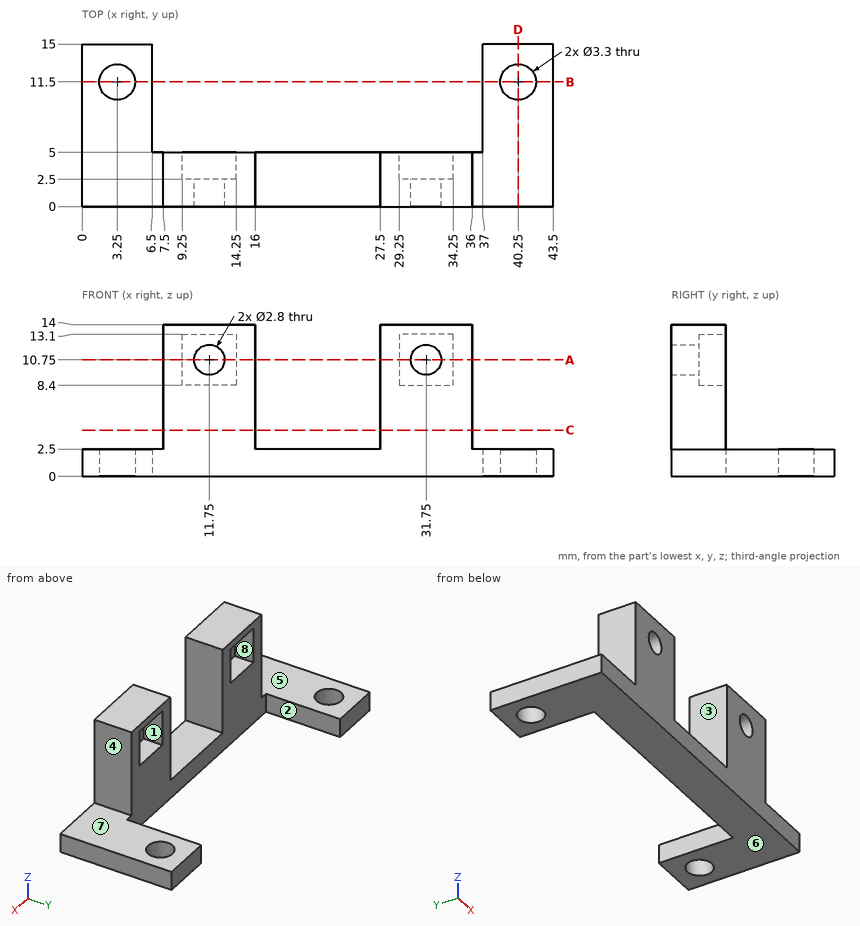
Verification items for this drawing (mm, ordinates from the low corner). A direction names the side the tool comes from. Give positions to 0.01 mm unless a question says otherwise; leave off trailing zeros. Write each loop counter-clockwise with the first axis right and the second up, starting at its lowest first coordinate (ties: lowest second). Pieces come first, ordered by that corner, then holes.
1) Gauge pin test, flat ends, axial feed: pin 1 (5.5 mm diameter, centred on y = 3, z = 10.5, fed in from -X); pin 2 (4.5 mm diameter, centred on x = 31.75, z = 10.75, fed in from +Y); pin 3 (4 mm diameter, centred on y = 2.5, z = 10.5, fed in from +X). Record the tip position at first contact, or that the pin passes through.
2) Section check A-A, the plane z = 10.75. Record the boundary of the cut face in (x, y).
3) Release check for a two-part mould opening along Z. For the marked faces 6, 7 and 8 record: pulls with the +Z half, pulls with the -Z half, needs draft (parallel to the pull), parting line crosses it, or undercut.
4) Material ranges on L1, parallel to X at y = 11.5, z = 0.8; L2, parallel to X at y = 4.75, z = 12; L3, parallel to Z at x = 31, y = 4.25, recorded low to high.
5) Section check C-C, the plane z = 4.25. Record the boundary of the cut face in (x, y), and give its area (3 significant figures).
6) Access from +Z, -Z, +X, -X, +Y, -Y to the whole of each face (thin tool, end or side, straight path). Record for the marked faces 1, 2, 3, 4 and 5.
7) Section check D-D, the plane x = 40.25. Record the boundary of the cut face in (y, z).
8) Section check B-B, the plane y = 11.5. Record the boundary of the cut face in (x, z), and give its area (3 significant figures).
Computed:
1. pin 1: stops at x = 7.5
1. pin 2: stops at y = 2.5
1. pin 3: stops at x = 36
2. outline: (7.5, 0) - (10.35, 0) - (10.35, 2.5) - (9.25, 2.5) - (9.25, 5) - (7.5, 5) - close; (13.15, 0) - (16, 0) - (16, 5) - (14.25, 5) - (14.25, 2.5) - (13.15, 2.5) - close; (27.5, 0) - (30.35, 0) - (30.35, 2.5) - (29.25, 2.5) - (29.25, 5) - (27.5, 5) - close; (33.15, 0) - (36, 0) - (36, 5) - (34.25, 5) - (34.25, 2.5) - (33.15, 2.5) - close
3. face 6: pulls with the -Z half
3. face 7: pulls with the +Z half
3. face 8: undercut
4. L1: x = 0 to 1.6, 4.9 to 6.5, 37 to 38.6, 41.9 to 43.5
4. L2: x = 7.5 to 9.25, 14.25 to 16, 27.5 to 29.25, 34.25 to 36
4. L3: z = 0 to 8.4, 13.1 to 14
5. outline: (7.5, 0) - (16, 0) - (16, 5) - (7.5, 5) - close; (27.5, 0) - (36, 0) - (36, 5) - (27.5, 5) - close
5. area: 85.0 mm2
6. face 1: +Y
6. face 2: +Z, -Z, +Y
6. face 3: +Z, +Y, -Y
6. face 4: +Z, +X, +Y, -Y
6. face 5: +Z, -X, +Y, -Y
7. outline: (0, 0) - (9.85, 0) - (9.85, 2.5) - (0, 2.5) - close; (13.15, 0) - (15, 0) - (15, 2.5) - (13.15, 2.5) - close
8. outline: (0, 0) - (1.6, 0) - (1.6, 2.5) - (0, 2.5) - close; (4.9, 0) - (6.5, 0) - (6.5, 2.5) - (4.9, 2.5) - close; (37, 0) - (38.6, 0) - (38.6, 2.5) - (37, 2.5) - close; (41.9, 0) - (43.5, 0) - (43.5, 2.5) - (41.9, 2.5) - close
8. area: 16.0 mm2
